Can you work these out from the model? Positions are in its coordinate system, mm. A direction names the side the tool comes from. Give positions to 0.01 mm unless a question says otherwise; leave off trailing zeros. Order: outer loops, then holes, each group sorted by start corner. A loop starts at its lowest first (then second) coordinate and runs counter-clockwise, first axis right, second up. Notation, with made-up numbers: M 41,-2 L 69,-2 A15 ccw 69,17 Z; hole C 83.5,80 d9. An arc over 180 degrees is marked long. Write each question's results on one line, items separated by ' | '.
from build123d import *

# Parameters (mm, degrees)
MAIN_DEPTH             = 80
SKETCH2_R              = 1.25
SKETCH2_R_2            = 1.5
MAKERBEAMFIXHOLE_DEPTH = 6.5
SKETCH3_W              = 2
SKETCH3_H              = 45
PINHOLES_DEPTH         = 2


with BuildPart() as part:
    # Sketch1 → Main (new body)
    with BuildSketch(Plane.XY):
        Polygon((-5, 0), (5, 0), (5, -4.5), (1.45, -4.5), (1.45, -5.5), (-1.45, -5.5), (-1.45, -4.5), (-5, -4.5), align=None)
    extrude(amount=MAIN_DEPTH)

    # Sketch2 → MakerBeamFixHole (cut, through all)
    with BuildSketch(Plane(origin=(0, 0, 0), x_dir=(1, 0, 0), z_dir=(0, 1, 0))):
        with Locations((0, -75)):
            Circle(SKETCH2_R)
        with Locations((0, -15)):
            Circle(SKETCH2_R)
        with Locations((0, -5)):
            Circle(SKETCH2_R_2)
    extrude(amount=-MAKERBEAMFIXHOLE_DEPTH, mode=Mode.SUBTRACT)

    # Sketch3 → PinHoles (cut)
    with BuildSketch(Plane(origin=(0, 0, 0), x_dir=(1, 0, 0), z_dir=(0, 1, 0))):
        with Locations((-4, -45)):
            Rectangle(SKETCH3_W, SKETCH3_H)
        with Locations((4, -45)):
            Rectangle(SKETCH3_W, SKETCH3_H)
    extrude(amount=-PINHOLES_DEPTH, mode=Mode.SUBTRACT)


solid = part.part
(1) Imagine slicing it at C-C, the plane y = -1. Write out the boundary of the cut face in (x, z), plus the area to 3 significant figures.
Data:
outline: M -5,0 L 5,0 L 5,22.5 L 3,22.5 L 3,67.5 L 5,67.5 L 5,80 L -5,80 L -5,67.5 L -3,67.5 L -3,22.5 L -5,22.5 Z; hole C 0,5 d3; hole C 0,15 d2.5; hole C 0,75 d2.5 | area: 603 mm2
(2) For faces 1 (the face through (3, -1, 45)), 2 (the face through (-4, -1, 22.5)), 3 (the face through (3, -4.5, 39)), which set-ups out of +Z, -Z, +X, -X, +Y, -Y let a thin tool reach every point of the face, with its end or its side?
Data:
face 1: +X, +Y | face 2: -X, +Y | face 3: +Z, -Z, +X, -Y
(3) We'd pull the mould along X, two halves only. Please class faces 4 (the face through (5, -3, 39)), 5 (the face through (-5, -3, 39)), 6 (the face through (-0.16, -2.71, 73.76)): +X half, -X half, draft (parallel to the pull), parting line (faces both ways), or undercut.
Data:
face 4: +X half | face 5: -X half | face 6: undercut
(4) Will these pins go through, and if not, where does the flat tip stop? P1, Ø1.1, axis at y = -5, z = 1.5, coming from the -X side; P2, Ø3, axis at x = 4, z = 40, coming from the -Y side; P3, Ø0.6, axis at y = -1.5, z = 41, coming from the -X side; P4, Ø1.6, axis at x = 4, z = 41.5, coming from the +Y side.
Data:
P1: stops at x = -5 | P2: stops at y = -4.5 | P3: stops at x = -3 | P4: stops at y = -2
(5) Imagine slicing it at A-A, the plane z = 15. Write out the boundary of the cut face in (x, y).
Data:
outline: M -5,-4.5 L -1.45,-4.5 L -1.45,-5.5 L -1.25,-5.5 L -1.25,0 L -5,0 Z; M 1.25,-5.5 L 1.45,-5.5 L 1.45,-4.5 L 5,-4.5 L 5,0 L 1.25,0 Z
(6) Imagine slicing it at B-B, the plane x = 0. Write out the boundary of the cut face in (y, z).
Data:
outline: M -5.5,0 L 0,0 L 0,3.5 L -5.5,3.5 Z; M -5.5,6.5 L 0,6.5 L 0,13.75 L -5.5,13.75 Z; M -5.5,16.25 L 0,16.25 L 0,73.75 L -5.5,73.75 Z; M -5.5,76.25 L 0,76.25 L 0,80 L -5.5,80 Z
(7) Imagine slicing it at D-D, the plane z = 27. Write out the boundary of the cut face in (x, y).
Data:
outline: M -5,-4.5 L -1.45,-4.5 L -1.45,-5.5 L 1.45,-5.5 L 1.45,-4.5 L 5,-4.5 L 5,-2 L 3,-2 L 3,0 L -3,0 L -3,-2 L -5,-2 Z
(8) I need wall thicknesses on L1, parallel to Z at x = 0, y = -2.15; L2, parallel to X at y = -1.6, z = 75; L3, parallel to X at y = -3.85, z = 5. Which ranges of each line are inside material? Lowest first, please. Write a range as from..to.
Data:
L1: z = 0..3.5, 6.5..13.75, 16.25..73.75, 76.25..80 | L2: x = -5..-1.25, 1.25..5 | L3: x = -5..-1.5, 1.5..5
